Geometry: final body of the model. Coordinates: model frame, mm. A direction names the side the tool comes from. Give positions to 0.01 mm unless a question says otherwise; leave off trailing zeros. Write each loop counter-clockwise with the first axis right and the second up, starting at its lowest first coordinate (ties: lowest second). Pieces come first, ordered by that corner, then holes.
Autodesk Inventor part; units mm, degrees
ref_plane "Work Plane1" through (0, 0, 0) normal (0, 0, 1) x (1, 0, 0)
ref_plane "YZ Plane" through (0, 0, 0) normal (1, 0, 0) x (0, 1, 0)
ref_plane "XZ Plane" through (0, 0, 0) normal (0, 1, 0) x (-1, 0, 0)
sketch "Sketch1: base" plane through (0, 0, 0) normal (0, 0, 1) x (1, 0, 0)
  circle A0 centre (-5, 4) radius 16.25
  circle A1 centre (-5, 4) radius 20.75
  circle A2 centre (-21, -12) radius 4.75
  circle A3 centre (11, -12) radius 4.75
  line L0 (-21, -12) -> (11, -12) construction
  line L1 (-21, 20) -> (-21, -12) construction
  point P0 (0, 0)
  point P1 (-5, -12)
  point P2 (-21, 4)
  point P3 (-22.3145, -7.4355)
  point P4 (-16.4355, -13.3145)
  point P5 (6.4355, -13.3145)
  point P6 (12.3145, -7.4355)
  dimension "d0" = 9.5
  dimension "d1" = 32
  dimension "d2" = 41.5
  dimension "d3" = 32.5
  dimension "d4" = 32
sketch "Sketch2: tube stopper" plane through (0, 0, 0) normal (0, 0, 1) x (1, 0, 0)
  circle A0 centre (-5, 4) radius 14.875
  circle A1 centre (-5, 4) radius 16.25
  point P0 (0, 0)
  dimension "d14" = 29.75
extrude "Ex1: base" add sketch "Sketch1: base" along normal blind 6
ref_plane "Work Plane1" through (0, 0, 0) normal (0, 0, 1) x (1, 0, 0)
sketch "Sketch: text" plane through (0, 0, 0) normal (0, 0, -1) x (-1, 0, 0)
  line L0 (3.25, 23.8) -> (6.75, 23.8) construction
  line L1 (6.75, 23.8) -> (6.75, 20.3) construction
  line L2 (6.75, 20.3) -> (3.25, 20.3) construction
  line L3 (3.25, 20.3) -> (3.25, 23.8) construction
  line L4 (2.1748, 22.7624) -> (3.0901, 22.7624)
  line L5 (3.0901, 22.7624) -> (3.5386, 21.3071)
  line L6 (3.5386, 21.3071) -> (3.9993, 22.7624)
  line L7 (3.9993, 22.7624) -> (4.8871, 22.7624)
  line L8 (4.8871, 22.7624) -> (3.9108, 20.465)
  line L9 (3.9108, 20.465) -> (3.1297, 20.465)
  line L10 (3.1297, 20.465) -> (2.1748, 22.7624)
  line L11 (5.0732, 23.635) -> (7.6422, 23.635)
  line L12 (7.6422, 23.635) -> (7.6422, 23.0401)
  spline S0 degree 2 poles (7.6422, 23.0401) (7.3066, 22.738) (7.0838, 22.3841) knots 0 0 0 1 1 1
  spline S1 degree 2 poles (7.0838, 22.3841) (6.8123, 21.9569) (6.6536, 21.4322) knots 0 0 0 1 1 1
  spline S2 degree 2 poles (6.6536, 21.4322) (6.5286, 21.0233) (6.4858, 20.465) knots 0 0 0 1 1 1
  line L13 (6.4858, 20.465) -> (5.6072, 20.465)
  spline S3 degree 2 poles (5.6072, 20.465) (5.7109, 21.24) (6.1563, 22.2926) (6.6384, 22.8906) knots 0 0 0 1 2 2 2
  line L14 (6.6384, 22.8906) -> (5.0732, 22.8906)
  line L15 (5.0732, 22.8906) -> (5.0732, 23.635)
  point P0 (0, 0)
  point P1 (5, 4)
  point P2 (5, 20.3)
  dimension "d22" = 3.5
  dimension "d23" = 16.3
hole "Hole1: M3 heat-sets" at (11, -12, 0) at (-21, -12, 0) direction (0, 0, -1) diameter 4.2 end through all both
extrude "Ex: tube stopper" [suppressed]
fillet "Fillet1" radius 2 2 edges at (12.3145, -7.4355, 3) (-22.3145, -7.4355, 3)
fillet "Fillet2" radius 1 5 edges at (-23.1529, -7.0697, 0) (-23.6764, -15.9242, 0) (13.1529, -7.0697, 0) (13.6764, -15.9242, 0) (-5, 24.75, 0)
extrude "Ex: text" cut sketch "Sketch: text" against normal blind 1 from surface at 0
properties part number "cage_inside_07"
Item 1: Section A-A, the plane y = 4. Return the cut outline in (x, z).
Found:
outline: (-25.75, 1) arc R1 ccw to (-24.75, 0) - (-21.25, 0) - (-21.25, 6) - (-25.75, 6) - close; (11.25, 0) - (14.75, 0) arc R1 ccw to (15.75, 1) - (15.75, 6) - (11.25, 6) - close
Item 2: Pin query (flat end, axial travel): pin 1 Ø0.8 at (y, z) = (23, 0.5) entering from -X; pin 2 Ø0.5 at (x, z) = (-3, 0.5) entering from -Y; pin 3 Ø1.5 at (y, z) = (7.5, 4) entering from -X. Return the tip coordinate at first contact, or that it passes through.
Found:
pin 1: stops at x = -13.99
pin 2: stops at y = -16.68
pin 3: stops at x = -25.57
Item 3: Line query: L1, parallel to Y at x = -5, z = 4.75; L2, parallel to X at y = 14.5, z = 4; L3, parallel to Y at x = -4.5, z = 0.5. Output: solid intervals per line, ascending.
Found:
L1: y = -16.75 to -12.25, 20.25 to 24.75
L2: x = -22.9 to -17.4, 7.4 to 12.9
L3: y = -16.74 to -12.24, 20.24 to 21.85, 22.76 to 24.61
Item 4: Pull-direction query (X, two-part tool) for faces 3 (the face through (-23.572, -15.994, 3.465)), 4 (the face through (-15, -10, 6)), 5 (the face through (-5.6, 24.74, 3.46)); classes: +X half, -X half, draft (parallel to the pull), parting line (faces both ways), or undercut.
Found:
face 3: undercut
face 4: draft
face 5: parting line
Item 5: Reachability of faces 1 (the face through (10.5, -0.88, 2.96)), 2 (the face through (-4.406, 21.63, 0.493)) from +Z, -Z, +X, -X, +Y, -Y: full face, straight path, thin tool, end or side. Return the list, or none.
Found:
face 1: +Z, -Z
face 2: -Z
Item 6: Section B-B, the plane z = 4.75. State how many separate pieces and enclosed holes the cut face has, plus the area to 3 significant figures.
Found:
separate pieces: 1
enclosed holes: 3
area: 605 mm2
